Part model, mm, in its own coordinate system. Coordinates: 2 decimals unless noted, no trailing zeros. Loops run counter-clockwise (first coordinate to the right, second up) from the corner with the lowest first, then second, coordinate; pieces in that order, holes last. Notation, with made-up numbers: (34.5, 48) - (73.5, 48) arc R36 cw to (73.5, 84) - close; hole circle Ø11 at (-11.75, 3.5). An arc over 180 degrees is marked (long way). Answer as CSV lines item,"result".
Autodesk Inventor part; units mm, degrees
ref_plane "YZ Plane" through (0, 0, 0) normal (1, 0, 0) x (0, 1, 0)
ref_plane "XZ Plane" through (0, 0, 0) normal (0, 1, 0) x (-1, 0, 0)
ref_plane "XY Plane" through (0, 0, 0) normal (0, 0, 1) x (1, 0, 0)
sketch "Эскиз1" plane through (0, 0, 0) normal (0, 1, 0) x (-1, 0, 0)
  line L0 (-5.5, -11.8) -> (-4.75, -11.8)
  circle A0 centre (-4.75, -8.8) radius 1.25
  circle A1 centre (-2.5, -23.8) radius 1.25
  circle A2 centre (-5.5, -19.8) radius 0.6
  circle A3 centre (-5.5, -21.8) radius 0.6
  circle A4 centre (-5.5, -17.8) radius 0.6
  circle A5 centre (-5.5, -15.8) radius 0.6
  circle A6 centre (-5.5, -13.8) radius 0.6
  circle A7 centre (-5.5, -11.8) radius 0.6
  line L1 (-0.5, -32.6) -> (-0.5, 0)
  line L2 (-0.5, -32.6) -> (-0.5, 0)
  line L3 (-0.5, 0) -> (-67.5, 0)
  line L4 (-67.5, 0) -> (-67.5, -32.6)
  line L5 (-67.5, -32.6) -> (-0.5, -32.6)
  line L6 (-0.5, -32.6) -> (-0.5, 0)
  dimension "d37" = 2.5
  dimension "d39" = 1.2
  dimension "d40" = 1.2
  dimension "d41" = 1.2
  dimension "d42" = 1.2
  dimension "d43" = 1.2
  dimension "d44" = 1.2
  dimension "d47" = 67
extrude "Выдавливание1" add sketch "Эскиз1" along normal blind 1
sketch "Эскиз2" plane through (0, 1, 0) normal (0, 1, 0) x (1, 0, 0)
  line L0 (0.5, 0) -> (67.5, 0)
  line L1 (0.5, 0) -> (0.5, 2)
  line L2 (0.5, 32.6) -> (0.5, 0)
  line L3 (0.5, 2) -> (67.5, 2)
  line L4 (67.5, 0) -> (67.5, 32.6)
  line L5 (0.5, 32.6) -> (0.5, 30.6)
  line L6 (0.5, 30.6) -> (67.5, 30.6)
  line L7 (67.5, 30.6) -> (68.5, 30.6)
  line L8 (68.5, 30.6) -> (68.5, 2)
  line L9 (68.5, 2) -> (67.5, 2)
  line L10 (67.5, 32.6) -> (0.5, 32.6)
  line L11 (0.5, 0) -> (67.5, 0)
  line L12 (67.5, 0) -> (67.5, 32.6)
  line L13 (67.5, 32.6) -> (0.5, 32.6)
  line L14 (0.5, 32.6) -> (0.5, 0)
  point P0 (0, 0)
  dimension "d48" = 2
  dimension "d49" = 2
  dimension "d50" = 1
extrude "Выдавливание2" cut sketch "Эскиз2" against normal blind 10 contours L1 L3 L4 L0 | L2 L10 L4 L6
sketch "Эскиз3" plane through (0, 1, 0) normal (0, 1, 0) x (1, 0, 0)
  line L0 (67.5, 2) -> (67.5, 30.6)
  line L1 (67.5, 2) -> (69.5, 2)
  line L2 (69.5, 2) -> (69.5, 30.6)
  line L3 (69.5, 30.6) -> (67.5, 30.6)
  line L4 (67.5, 30.6) -> (67.5, 2)
  point P0 (0, 0)
  dimension "d53" = 2
extrude "Выдавливание3" add sketch "Эскиз3" against normal blind 1
properties part number "akkum_board"
Q1. Saw through at B-B (z = -8.8). Give the cut face in (x, y), then the cut area to 3 significant figures.
Results:
outline,"(0.5, 0) - (3.5, 0) - (3.5, 1) - (0.5, 1) - close; (6, 0) - (69.5, 0) - (69.5, 1) - (6, 1) - close"
area,"66.5 mm^2"
Q2. Wall check: L1, parallel to X at y = 0.2, z = -23. Give the ranges that are in metal, low to high.
Results:
L1,"x = 0.5 to 1.54, 3.46 to 69.5"
Q3. Saw through at A-A (x = 2.5). Give the cut face in (y, z).
Results:
outline,"(0, -30.6) - (1, -30.6) - (1, -25.05) - (0, -25.05) - close; (0, -22.55) - (1, -22.55) - (1, -2) - (0, -2) - close"
Q4. Flat gauge pin, fed straight in: pin 1 (1.5 mm diameter, centred on x = 2.5, z = -23.8, fed in from +Y). Where does the tip first touch, or does it go through?
Results:
pin 1,"passes through"
